The listing builds one solid part. Answer for the finished solid, in the listing's coordinates (mm). A direction names the side the tool comes from. Give positions to 0.01 mm unless a question says otherwise; leave off trailing zeros. Order: outer loops, then holes, each group sorted by start corner. A loop starts at its lowest first (then second) coordinate and runs counter-clockwise, first axis right, second up. Notation, with made-up numbers: (63.5, 22) - (83.5, 22) arc R33 ccw to (83.5, 57) - close; hole circle Ø9 at (-27, -36.75). An arc over 180 degrees is marked (long way). Use CSV: the item, a comma, the result in double quotes.
```python
from build123d import *

# Parameters (mm, degrees)
F1_DEPTH       = 50
F3_DEPTH       = 8
F5_D           = 6.6
F5_CBORE_D     = 11.25
F5_CBORE_DEPTH = 6
F7_D           = 3.3
F8_DEPTH       = 15


with BuildPart() as f1:
    # F0 (on Front) → F1 (new body)
    with BuildSketch(Plane.XZ):
        Polygon((0, -30), (0, 0), (-4, 0), (-4, -11), (-17, -11), (-17, 0), (-40, 0), (-40, -30), align=None)
    extrude(amount=F1_DEPTH)

    # F2 (on face) → F3 (cut)
    with BuildSketch(Plane.XY):
        Polygon((-40, -16), (-40, -25), (-40, -34), (-17, -34), (-17, -16), align=None)
    extrude(amount=-F3_DEPTH, mode=Mode.SUBTRACT)

    # F5 (through all)
    with Locations(Plane.XY):
        with Locations((-30, -40)):
            CounterBoreHole(F5_D / 2, F5_CBORE_D / 2, F5_CBORE_DEPTH)

    # F7 (through all)
    with Locations(Plane.XY):
        with Locations((-30, -8)):
            Hole(F7_D / 2)

    # F8 (cut): a face of the model
    f8_faces = [f1.faces().sort_by_distance(p)[0] for p in [
        (-19.7815033531, -24.8120928837, -30),
    ]]
    extrude(f8_faces, amount=-F8_DEPTH, mode=Mode.SUBTRACT)


solid = f1.part
```
Item 1: The part is cut by section B-B (y = -8). Give the vertices of the cut face in (x, z), and give its area (4 significant figures).
Taken from the geometry:
outline,"(-40, -15) - (-31.65, -15) - (-31.65, 0) - (-40, 0) - close; (-28.35, -15) - (0, -15) - (0, 0) - (-4, 0) - (-4, -11) - (-17, -11) - (-17, 0) - (-28.35, 0) - close"
area,"407.5 mm^2"
Item 2: The part is cut by section C-C (x = -30). Give the vertices of the cut face in (y, z) (3 decimals), and give its area (3 significant figures).
Taken from the geometry:
outline,"(-50, -15) - (-43.3, -15) - (-43.3, -6) - (-45.625, -6) - (-45.625, 0) - (-50, 0) - close; (-36.7, -15) - (-9.65, -15) - (-9.65, 0) - (-16, 0) - (-16, -8) - (-34, -8) - (-34, 0) - (-34.375, 0) - (-34.375, -6) - (-36.7, -6) - close; (-6.35, -15) - (0, -15) - (0, 0) - (-6.35, 0) - close"
area,"430 mm^2"
Item 3: Each of these flat-tipped pins is pushed along its axis until it touches: pin 1 (8.5 mm diameter, centred on x = -30, y = -40, fed in from +Z); pin 2 (10 mm diameter, centred on x = -9.5, y = -26, fed in from +Z); pin 3 (2.5 mm diameter, centred on x = -30, y = -8, fed in from +Z); pin 4 (5.5 mm diameter, centred on x = -29, y = -23, fed in from +Z). Where does it stop, or does it pass through?
Taken from the geometry:
pin 1,"z = -6"
pin 2,"z = -11"
pin 3,"through"
pin 4,"z = -8"
Item 4: The mould has two halves that part along X. Classify faces 4 (the face through (-30.732, -34.423, -2.958)), 5 (the face through (0, -25, -8)), 6 (the face through (-2, -25, 0)): +X half, -X half, draft (parallel to the pull), parting line (faces both ways), or undercut.
Taken from the geometry:
face 4,"undercut"
face 5,"+X half"
face 6,"draft"
Item 5: The part is cut by section A-A (z = -2.5). Give the vertices of the cut face in (x, y) (3 decimals), and give its area (3 significant figures).
Taken from the geometry:
outline,"(-40, -50) - (-17, -50) - (-17, -34) - (-40, -34) - close; (-40, -16) - (-17, -16) - (-17, 0) - (-40, 0) - close; (-4, -50) - (0, -50) - (0, 0) - (-4, 0) - close; hole circle Ø11.25 at (-30, -40); hole circle Ø3.3 at (-30, -8)"
area,"828 mm^2"
Item 6: Which of the six approach directions +Z, -Z, +X, -X, +Y, -Y give full straight-line access (tool end or side, diameter ignored) to faces 1 (the face through (-17, -25, -9)), 2 (the face through (-29, -34, -4)), 3 (the face through (-30, -44, -6))?
Taken from the geometry:
face 1,"+Z, +Y, -Y"
face 2,"+Z, -X"
face 3,"+Z"
Item 7: Find the intervals of material crossed by line 1 along Y through (x, z) = (-30, -8.75); line 2 along Y through (x, z) = (-30, -3.15) (3 decimals); line 3 along X through (y, z) = (-12.5, -8.25), in increasing order.
Taken from the geometry:
line 1,"-50 to -43.3, -36.7 to -9.65, -6.35 to 0"
line 2,"-50 to -45.625, -34.375 to -34, -16 to -9.65, -6.35 to 0"
line 3,"-40 to -17, -4 to 0"
Item 8: The part is cut by section D-D (y = -47). Give the vertices of the cut face in (x, z), and give its area (3 significant figures).
Taken from the geometry:
outline,"(-40, -15) - (0, -15) - (0, 0) - (-4, 0) - (-4, -11) - (-17, -11) - (-17, 0) - (-40, 0) - close"
area,"457 mm^2"
